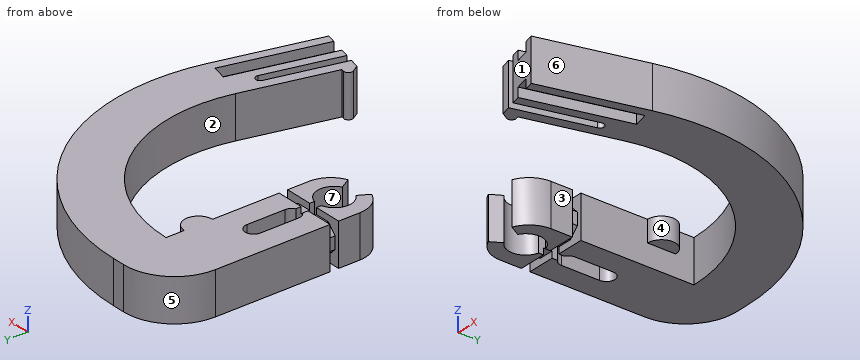
from build123d import *

# Parameters (mm, degrees)
SKETCH003_W          = 7.5
SKETCH003_H          = 26
PAD_DEPTH            = 2.5
SKETCH004_R          = 1.65
PAD001_DEPTH         = 2.5
FILLET_R             = 6
SKETCH005_R          = 2
POCKET_DEPTH         = 2.501
POCKET_DEPTH_BACK    = 2.501
SKETCH006_W          = 1
SKETCH006_H          = 5
POCKET001_DEPTH      = 2.501
POCKET001_DEPTH_BACK = 2.501
POCKET002_DEPTH      = 58.526798
POCKET002_DEPTH_BACK = 58.526798
SKETCH009_W          = 7.5
SKETCH009_H          = 5
POCKET003_DEPTH      = 0.5
PAD002_DEPTH         = 2.5
POCKET004_DEPTH      = 2.501
POCKET004_DEPTH_BACK = 2.501
PAD003_DEPTH         = 2.5
POCKET005_DEPTH      = 1.1


with BuildPart() as part:
    # Sketch003 → Pad (new body, symmetric)
    with BuildSketch(Plane.XY):
        with Locations((0, 13)):
            Rectangle(SKETCH003_W, SKETCH003_H)
    extrude(amount=PAD_DEPTH, both=True)

    # Sketch004 → Pad001 (join)
    with BuildSketch(Plane.XY):
        with Locations((3.75, 16)):
            Circle(SKETCH004_R)
    extrude(amount=PAD001_DEPTH)

    # Fillet
    fillet_edges = [part.edges().sort_by_distance(p)[0] for p in [
        (-3.75, 26, 0),
    ]]
    fillet(fillet_edges, radius=FILLET_R)

    # Sketch005 → Pocket (cut, two sides)
    with BuildSketch(Plane.XY) as pocket_sk:
        with Locations((0, 3)):
            Circle(SKETCH005_R)
        with BuildLine():
            ThreePointArc((1, 12.5), (0, 13.5), (-1, 12.5))
            Line((-1, 12.5), (-1, 8))
            ThreePointArc((-1, 8), (0, 7), (1, 8))
            Line((1, 8), (1, 12.5))
        make_face()
    extrude(amount=-POCKET_DEPTH, mode=Mode.SUBTRACT)
    extrude(pocket_sk.sketch, amount=POCKET_DEPTH_BACK, mode=Mode.SUBTRACT)

    # Sketch006 → Pocket001 (cut, two sides)
    with BuildSketch(Plane.XY) as pocket001_sk:
        Polygon((-1.732051, 0), (0, 3), (1.732051, 0), align=None)
        with Locations((0, 5.5)):
            Rectangle(SKETCH006_W, SKETCH006_H)
    extrude(amount=-POCKET001_DEPTH, mode=Mode.SUBTRACT)
    extrude(pocket001_sk.sketch, amount=POCKET001_DEPTH_BACK, mode=Mode.SUBTRACT)

    # Sketch007 → Pocket002 (cut, two sides)
    with BuildSketch(Plane.XY) as pocket002_sk:
        with BuildLine():
            ThreePointArc((1.732051, 0), (3.198765, 1.196569), (3.75, 3.007416))
            Line((3.75, 0), (3.75, 3.007416))
            Line((1.732051, 0), (3.75, 0))
        make_face()
    pocket002 = extrude(amount=-POCKET002_DEPTH, mode=Mode.SUBTRACT) + extrude(pocket002_sk.sketch, amount=POCKET002_DEPTH_BACK, mode=Mode.SUBTRACT)

    # Mirrored: Pocket002 across YZ
    add(pocket002.mirror(Plane.YZ), mode=Mode.SUBTRACT)

    # Sketch009 → Pocket003 (cut, symmetric)
    with BuildSketch(Plane.XZ.offset(-6)):
        Rectangle(SKETCH009_W, SKETCH009_H)
        Polygon((-2.224874, 1.75), (-3.25, 0.724874), (-3.25, -0.724874), (-2.224874, -1.75), (2.224874, -1.75), (3.25, -0.724874), (3.25, 0.724874), (2.224874, 1.75), align=None, mode=Mode.SUBTRACT)
    extrude(amount=POCKET003_DEPTH, both=True, mode=Mode.SUBTRACT)

    # Sketch010 → Pad002 (join, symmetric)
    with BuildSketch(Plane.XY):
        with BuildLine():
            ThreePointArc((26.768892, -3.462839), (22.44444, 16.882113), (3.75, 26))
            Line((3.75, 19.8), (3.75, 26))
            ThreePointArc((20.753059, -1.962923), (17.558773, 13.065011), (3.75, 19.8))
            Line((20.753059, -1.962923), (17.784166, -13.8705))
            Line((17.784166, -13.8705), (23.8, -15.370416))
            Line((23.8, -15.370416), (26.768892, -3.462839))
        make_face()
    extrude(amount=PAD002_DEPTH, both=True)

    # Sketch011 → Pocket004 (cut, two sides)
    with BuildSketch(Plane.XY) as pocket004_sk:
        with BuildLine():
            ThreePointArc((18.948521, -14.160807), (19.312708, -14.766915), (19.918817, -14.402728))
            Line((19.918817, -14.402728), (22.096114, -5.670067))
            ThreePointArc((22.096114, -5.670067), (21.731927, -5.063958), (21.125818, -5.428145))
            Line((21.125818, -5.428145), (18.948521, -14.160807))
        make_face()
    extrude(amount=-POCKET004_DEPTH, mode=Mode.SUBTRACT)
    extrude(pocket004_sk.sketch, amount=POCKET004_DEPTH_BACK, mode=Mode.SUBTRACT)

    # Sketch012 → Pad003 (join, symmetric)
    with BuildSketch(Plane.XY):
        with BuildLine():
            Line((17.784166, -13.8705), (18.148769, -12.408161))
            Line((18.148769, -12.408161), (17.85768, -12.335584))
            ThreePointArc((17.85768, -12.335584), (17.334791, -12.523321), (17.308135, -13.078251))
            Line((17.308135, -13.078251), (17.784166, -13.8705))
        make_face()
    extrude(amount=PAD003_DEPTH, both=True)

    # Sketch013 → Pocket005 (cut)
    with BuildSketch(Plane.XY.offset(2.5)):
        Polygon((20.986142, -14.668843), (23.889205, -3.025294), (25.635737, -3.460753), (22.732675, -15.104302), align=None)
    pocket005 = extrude(amount=-POCKET005_DEPTH, mode=Mode.SUBTRACT)

    # Mirrored001: Pocket005 across XY
    add(pocket005.mirror(Plane.XY), mode=Mode.SUBTRACT)


solid = part.part
Design review of the part built by this model. Coordinates are the model's own, in mm. Face numbers are marked on the shaded views. A direction names the side the tool comes from. Give positions to 0.01 mm unless a question says otherwise; leave off trailing zeros. Order: outer loops, then holes, each group sorted by start corner. A loop starts at its lowest first (then second) coordinate and runs counter-clockwise, first axis right, second up. Notation, with made-up numbers: (-6.75, 68.25) - (32.25, 68.25) arc R26 cw to (32.25, 91.25) - close; hole circle Ø10 at (4.5, 46.5). An arc over 180 degrees is marked (long way). Write item = value, one per line. Start each with the question number.
Q1. To check wall thickness, follow L1, parallel to X at y = 5, z = -1.8; L2, parallel to X at y = 1, z = 1.65; L3, parallel to Y at x = -1.5, z = 2.25. State the ranges of each line that lie inside material, in increasing order. Write a range as from..to.
Q2. Mouldability with a two-part tool opening along Y and no side actions: class the marked faces 4, 5, 6 and 7 as released by +Y, released by -Y, zero draft, split by the parting line, or undercut.
Q3. Clearance check with flat-ended pins moving along their axes: pin 1 Ø1 at (x, z) = (8.5, -1) entering from -Y; pin 2 Ø2 at (y, z) = (11.5, 0.5) entering from +X; pin 3 Ø1 at (x, z) = (-2.5, 0.5) entering from -Y. State where each tip first meets the part, or that it passes through.
Q4. We need section C-C on y = -1. State the section outline as (x, z) points, plus the area to 3 significant figures.
Q5. We need section B-B on x = 8.5. State the section outline as (y, z) points.
Q6. Tool access review of the marked faces 1, 2 and 3: name each direction out of +Z, -Z, +X, -X, +Y, -Y from which nothing blocks a thin tool from reaching the whole face with its end or side.
Q7. We need section A-A on y = 13. State the section outline as (x, z) points.
Working result:
q1.L1 = -3.75..-0.5, 0.5..3.75, 21.06..27.32
q1.L2 = -3.06..-1.15, 1.15..3.06, 21.23..27.44
q1.L3 = 0.4..1.68, 4.32..5.5, 6.5..24.68
q2.face_4 = undercut
q2.face_5 = released by +Y
q2.face_6 = released by -Y
q2.face_7 = undercut
q3.pin_1 = 19
q3.pin_2 = 26
q3.pin_3 = 0.12
q4.outline = (20.96, -2.5) - (27.25, -2.5) - (27.25, 2.5) - (20.96, 2.5) - close
q4.area = 31.4 mm²
q5.outline = (19.14, -2.5) - (25.52, -2.5) - (25.52, 2.5) - (19.14, 2.5) - close
q6.face_1 = +Z, -Z, -X, -Y
q6.face_2 = +Z, -Z
q6.face_3 = +Z, -Z, -Y
q7.outline = (-3.75, -2.5) - (-0.87, -2.5) - (-0.87, 2.5) - (-3.75, 2.5) - close; (0.87, -2.5) - (3.75, -2.5) - (3.75, 2.5) - (0.87, 2.5) - close; (17.61, -2.5) - (24.91, -2.5) - (24.91, 2.5) - (17.61, 2.5) - close
